from build123d import *

# Parameters (mm, degrees)
SKETCH1_W           = 20
SKETCH1_H           = 90.600658981
BOSS_EXTRUDE1_DEPTH = 3
FILLET1_R           = 3


with BuildPart() as part:
    # Sketch1 → Boss-Extrude1 (new body)
    with BuildSketch(Plane.XY):
        with Locations((-91.066816784, 79.208884685)):
            Rectangle(SKETCH1_W, SKETCH1_H)
        with BuildLine():
            Line((-86.19596438, 38.053580074), (-95.937669189, 38.053580074))
            ThreePointArc((-95.937669189, 38.053580074), (-97.965327886, 40.081238771), (-95.937669189, 42.108897468))
            Line((-95.937669189, 42.108897468), (-86.19596438, 42.108897468))
            ThreePointArc((-86.19596438, 42.108897468), (-84.168305683, 40.081238771), (-86.19596438, 38.053580074))
        make_face(mode=Mode.SUBTRACT)
        with BuildLine():
            Line((-86.19596438, 48.053580074), (-95.937669189, 48.053580074))
            ThreePointArc((-95.937669189, 48.053580074), (-97.965327886, 50.081238771), (-95.937669189, 52.108897468))
            Line((-95.937669189, 52.108897468), (-86.19596438, 52.108897468))
            ThreePointArc((-86.19596438, 52.108897468), (-84.168305683, 50.081238771), (-86.19596438, 48.053580074))
        make_face(mode=Mode.SUBTRACT)
        with BuildLine():
            Line((-86.19596438, 58.053580074), (-95.937669189, 58.053580074))
            ThreePointArc((-95.937669189, 58.053580074), (-97.965327886, 60.081238771), (-95.937669189, 62.108897468))
            Line((-95.937669189, 62.108897468), (-86.19596438, 62.108897468))
            ThreePointArc((-86.19596438, 62.108897468), (-84.168305683, 60.081238771), (-86.19596438, 58.053580074))
        make_face(mode=Mode.SUBTRACT)
        with BuildLine():
            Line((-86.19596438, 68.053580074), (-95.937669189, 68.053580074))
            ThreePointArc((-95.937669189, 68.053580074), (-97.965327886, 70.081238771), (-95.937669189, 72.108897468))
            Line((-95.937669189, 72.108897468), (-86.19596438, 72.108897468))
            ThreePointArc((-86.19596438, 72.108897468), (-84.168305683, 70.081238771), (-86.19596438, 68.053580074))
        make_face(mode=Mode.SUBTRACT)
        with BuildLine():
            Line((-86.19596438, 78.053580074), (-95.937669189, 78.053580074))
            ThreePointArc((-95.937669189, 78.053580074), (-97.965327886, 80.081238771), (-95.937669189, 82.108897468))
            Line((-95.937669189, 82.108897468), (-86.19596438, 82.108897468))
            ThreePointArc((-86.19596438, 82.108897468), (-84.168305683, 80.081238771), (-86.19596438, 78.053580074))
        make_face(mode=Mode.SUBTRACT)
        with BuildLine():
            Line((-86.19596438, 88.053580074), (-95.937669189, 88.053580074))
            ThreePointArc((-95.937669189, 88.053580074), (-97.965327886, 90.081238771), (-95.937669189, 92.108897468))
            Line((-95.937669189, 92.108897468), (-86.19596438, 92.108897468))
            ThreePointArc((-86.19596438, 92.108897468), (-84.168305683, 90.081238771), (-86.19596438, 88.053580074))
        make_face(mode=Mode.SUBTRACT)
        with BuildLine():
            Line((-86.19596438, 98.053580074), (-95.937669189, 98.053580074))
            ThreePointArc((-95.937669189, 98.053580074), (-97.965327886, 100.081238771), (-95.937669189, 102.108897468))
            Line((-95.937669189, 102.108897468), (-86.19596438, 102.108897468))
            ThreePointArc((-86.19596438, 102.108897468), (-84.168305683, 100.081238771), (-86.19596438, 98.053580074))
        make_face(mode=Mode.SUBTRACT)
        with BuildLine():
            Line((-86.19596438, 108.053580074), (-95.937669189, 108.053580074))
            ThreePointArc((-95.937669189, 108.053580074), (-97.965327886, 110.081238771), (-95.937669189, 112.108897468))
            Line((-95.937669189, 112.108897468), (-86.19596438, 112.108897468))
            ThreePointArc((-86.19596438, 112.108897468), (-84.168305683, 110.081238771), (-86.19596438, 108.053580074))
        make_face(mode=Mode.SUBTRACT)
        with BuildLine():
            Line((-86.19596438, 118.053580074), (-95.937669189, 118.053580074))
            ThreePointArc((-95.937669189, 118.053580074), (-97.965327886, 120.081238771), (-95.937669189, 122.108897468))
            Line((-95.937669189, 122.108897468), (-86.19596438, 122.108897468))
            ThreePointArc((-86.19596438, 122.108897468), (-84.168305683, 120.081238771), (-86.19596438, 118.053580074))
        make_face(mode=Mode.SUBTRACT)
    extrude(amount=BOSS_EXTRUDE1_DEPTH)

    # Fillet1
    fillet1_edges = [part.edges().sort_by_distance(p)[0] for p in [
        (-101.066816784, 124.509214175, 1.5),
        (-81.066816784, 124.509214175, 1.5),
        (-81.066816784, 33.908555194, 1.5),
        (-101.066816784, 33.908555194, 1.5),
    ]]
    fillet(fillet1_edges, radius=FILLET1_R)


solid = part.part
For this review, take the finished solid that the model builds, in its own axes (mm). A direction names the side the tool comes from. Round coordinates to 2 decimals unless told otherwise and drop trailing zeros. Loops run counter-clockwise (first coordinate to the right, second up) from the corner with the lowest first, then second, coordinate; pieces in that order, holes last. Notation, with made-up numbers: (-27, 69.25) - (-16, 69.25) arc R19 cw to (-16, 93.25) - close; hole circle Ø4 at (2.25, 79.25). An arc over 180 degrees is marked (long way). Use one line per item in the form item = value.
1) We need section A-A on y = 70.5. Write out the cut boundary in (x, z).
Solutions:
outline = (-101.07, 0) - (-97.92, 0) - (-97.92, 3) - (-101.07, 3) - close; (-84.21, 0) - (-81.07, 0) - (-81.07, 3) - (-84.21, 3) - close
2) Mouldability with a two-part tool opening along X and no side actions: class faces 1 (the face through (-91, 48.054, 1)), 2 (the face through (-91, 124.509, 1)), 3 (the face through (-100.2, 34.8, 1.5)) as pulls with the +X half, pulls with the -X half, needs draft (parallel to the pull), parting line crosses it, or undercut.
Solutions:
face_1 = undercut
face_2 = needs draft
face_3 = pulls with the -X half
3) Wall thickness on probe 1 along X at (y, z) = (40.5, 2.5); probe 2 along X at (y, z) = (79, 0.6): over which ranges is each line inside the solid? List them lowest first.
Solutions:
probe_1 = -101.07 to -97.92, -84.21 to -81.07
probe_2 = -101.07 to -97.65, -84.48 to -81.07
4) Tool access review of faces 4 (the face through (-101.067, 79, 1)), 5 (the face through (-97.965, 60.037, 1.479)): name each direction out of +Z, -Z, +X, -X, +Y, -Y from which nothing blocks a thin tool from reaching the whole face with its end or side.
Solutions:
face_4 = +Z, -Z, -X, +Y, -Y
face_5 = +Z, -Z
5) We need section D-D on y = 89.5. Write out the cut boundary in (x, z), then the cut area to 3 significant figures.
Solutions:
outline = (-101.07, 0) - (-97.88, 0) - (-97.88, 3) - (-101.07, 3) - close; (-84.25, 0) - (-81.07, 0) - (-81.07, 3) - (-84.25, 3) - close
area = 19.1 mm2
6) We need section B-B on x = -88. State how many separate pieces and enclosed holes the cut face has, then the cut area to 3 significant figures.
Solutions:
separate_pieces = 10
enclosed_holes = 0
area = 162 mm2
